Part print with two shaded views. Sizes in mm from the minimum x, y, z corner. A direction names the side the tool comes from. Round coordinates to 2 decimals unless told otherwise and drop trailing zeros. Loops run counter-clockwise (first coordinate to the right, second up) from the corner with the lowest first, then second, coordinate; pieces in that order, holes last. Notation, with made-up numbers: M 81.25,35 L 133.25,35 A11 cw 133.25,44 Z; hole C 59.5,3 d6. An arc over 180 degrees is marked long. Use a Markdown table: item, result. Add a question column.
Item 1: Tool access for the marked faces 1, 2 and 3: list every direction of +Z, -Z, +X, -X, +Y, -Y with a clear straight run to the whole face (end or side of a thin tool).
Item 2: Pin check, flat tips, straight feed: P1, Ø12, axis at x = 39, y = 66.5, coming from the +Z side; P2, Ø11, axis at x = 16.5, z = 39, coming from the -Y side (3 decimals); P3, Ø6.5, axis at x = 18.5, z = 42.5, coming from the +Y side (3 decimals). Stop position of each tip, or through.
Item 3: Saw through at D-D on x = 16. Write the cut outline in (y, z) (3 decimals), then the cut area to 3 significant figures.
Item 4: Saw through at C-C on y = 62. Write the cut outline in (x, z) (3 decimals), then the cut area to 3 significant figures.
Item 5: Saw through at B-B on z = 21. Write the cut outline in (x, y) (3 decimals), then the cut area to 3 significant figures.
Item 6: Wall check: L1, parallel to X at y = 5.5, z = 36.5 (3 decimals); L2, parallel to Y at x = 15.5, z = 36.5 (3 decimals); L3, parallel to Z at x = 46.5, y = 60.5. Give the ranges that are in metal, low to high. Write a range as from..to.
Item 7: Saw through at A-A on x = 27. Write the cut outline in (y, z) (3 decimals), then the cut area to 3 significant figures.
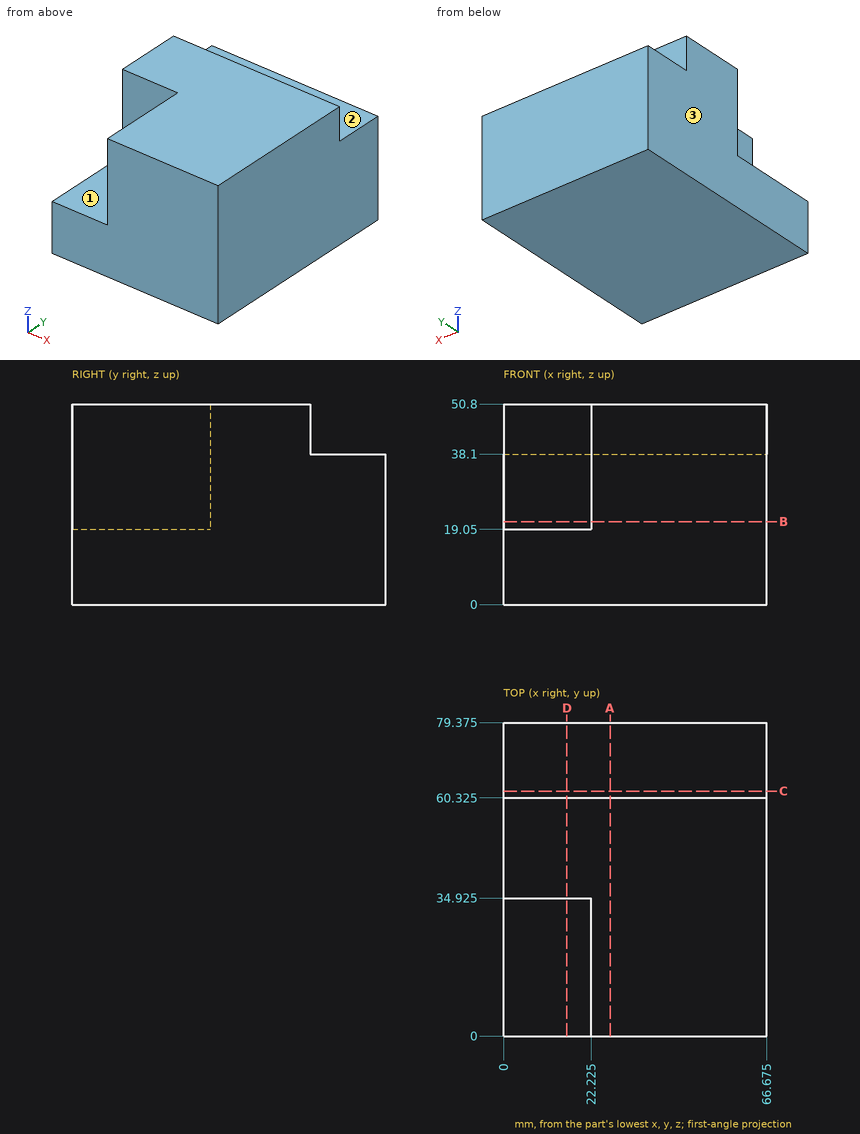
Entries:
| question | item | result |
|---|---|---|
| 1 | face 1 | +Z, -X, -Y |
| 1 | face 2 | +Z, +X, -X, +Y |
| 1 | face 3 | +Z, -Z, -X, +Y, -Y |
| 2 | P1 | z = 38.1 |
| 2 | P2 | y = 34.925 |
| 2 | P3 | y = 60.325 |
| 3 | outline | M 0,0 L 79.375,0 L 79.375,38.1 L 60.325,38.1 L 60.325,50.8 L 34.925,50.8 L 34.925,19.05 L 0,19.05 Z |
| 3 | area | 2,680 mm2 |
| 4 | outline | M 0,0 L 66.675,0 L 66.675,38.1 L 0,38.1 Z |
| 4 | area | 2,540 mm2 |
| 5 | outline | M 0,34.925 L 22.225,34.925 L 22.225,0 L 66.675,0 L 66.675,79.375 L 0,79.375 Z |
| 5 | area | 4,520 mm2 |
| 6 | L1 | 22.225..66.675 |
| 6 | L2 | 34.925..79.375 |
| 6 | L3 | 0..38.1 |
| 7 | outline | M 0,0 L 79.375,0 L 79.375,38.1 L 60.325,38.1 L 60.325,50.8 L 0,50.8 Z |
| 7 | area | 3,790 mm2 |
